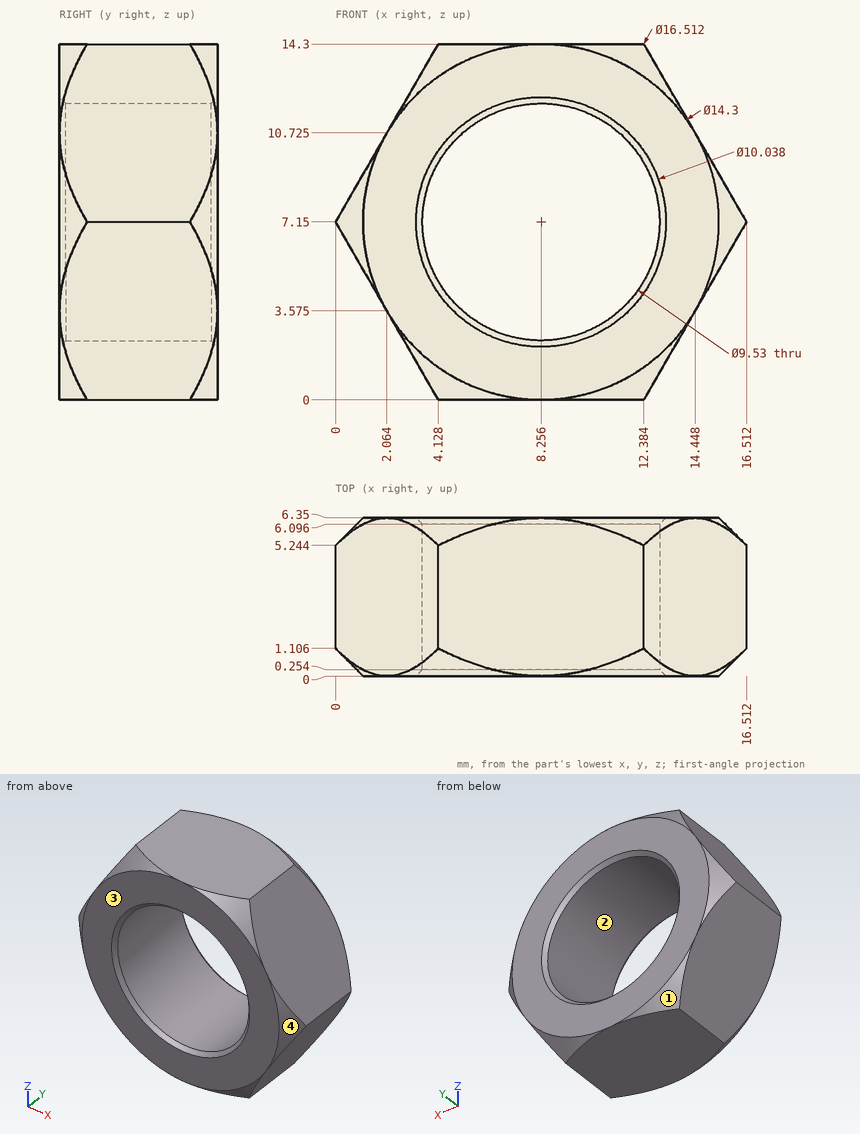
Here's the drawing with two shaded views (mm, measured from the low corner). I have some questions. Coordinates: 2 decimals unless noted, no trailing zeros.
Item 1: If we mould it in two halves opening along X, with no side actions, what happens to the marked faces 1, 2, 3 and 4? For each: +X half, -X half, draft (parallel to the pull), parting line (faces both ways), or undercut.
Result sheet:
face 1: -X half
face 2: undercut
face 3: draft
face 4: +X half
Item 2: For P1, Ø2, axis at y = 5.5, z = 3.5, coming from the -X side; P2, Ø1, axis at x = 2, y = 3, coming from the +Z side; P3, Ø2, axis at y = 3.5, z = 3, coming from the -X side, each with a flat end and sliding along its axis, tell me the tip position at first contact or that it passes through.
Result sheet:
P1: stops at x = 1.53
P2: stops at z = 11.48
P3: stops at x = 1.82
Item 3: I need wall thicknesses on line 1 (Z direction, x = 11.75, y = 4); line 2 (X direction, y = 3, z = 9.5) (1 decimal); line 3 (X direction, y = 6, z = 3.5) (1 decimal). Which ranges of each line are inside material? Lowest first, please.
Result sheet:
line 1: z = 0 to 3.91, 10.39 to 14.3
line 2: x = 1.4 to 4.1, 12.4 to 15.2
line 3: x = 2.1 to 5.2, 11.3 to 14.4
